from build123d import *

# Parameters (mm, degrees)
SKETCH1_R           = 2.54
BOSS_EXTRUDE1_DEPTH = 3.81
SKETCH2_R           = 4.953
BOSS_EXTRUDE2_DEPTH = 76.2
FILLET1_R           = 2.54


with BuildPart() as part:
    # Sketch1 → Boss-Extrude1 (new body)
    with BuildSketch(Plane(origin=(0, 0, 0), x_dir=(1, 0, 0), z_dir=(0, 1, 0))):
        with BuildLine():
            Line((-13.97, -6.985), (13.97, -6.985))
            ThreePointArc((13.97, -6.985), (15.766051224, -6.241051224), (16.51, -4.445))
            Line((16.51, -4.445), (16.51, 4.445))
            ThreePointArc((16.51, 4.445), (15.766051224, 6.241051224), (13.97, 6.985))
            Line((13.97, 6.985), (-13.97, 6.985))
            ThreePointArc((-13.97, 6.985), (-15.766051224, 6.241051224), (-16.51, 4.445))
            Line((-16.51, 4.445), (-16.51, -4.445))
            ThreePointArc((-16.51, -4.445), (-15.766051224, -6.241051224), (-13.97, -6.985))
        make_face()
        with Locations(Location((-12.7, 0, 0), (0, 0, 90))):
            Circle(SKETCH1_R, mode=Mode.SUBTRACT)
        with Locations(Location((12.7, 0, 0), (0, 0, 90))):
            Circle(SKETCH1_R, mode=Mode.SUBTRACT)
    extrude(amount=BOSS_EXTRUDE1_DEPTH)

    # Sketch2 → Boss-Extrude2 (add)
    with BuildSketch(Plane(origin=(0, 3.81, 0), x_dir=(1, 0, 0), z_dir=(0, 1, 0))):
        with Locations(Location((0, 0, 0), (0, 0, 90))):
            Circle(SKETCH2_R)
    extrude(amount=BOSS_EXTRUDE2_DEPTH)

    # Fillet1
    fillet1_edges = [part.edges().sort_by_distance(p)[0] for p in [
        (0, 3.81, 4.953),
    ]]
    fillet(fillet1_edges, radius=FILLET1_R)


solid = part.part
Verification items for the finished model (mm, model axes). A direction names the side the tool comes from. Coordinates: 2 decimals unless noted, no trailing zeros. Write each loop counter-clockwise with the first axis right and the second up, starting at its lowest first coordinate (ties: lowest second). Pieces come first, ordered by that corner, then holes. Notation, with made-up numbers: M 88.5,7 L 110.5,7 A19 ccw 110.5,35 Z; hole C 77,-9 d5. An arc over 180 degrees is marked long. One line per question, with ' | ' between items.
1) Depth check by flat-ended pin: pin 1 Ø6 at (x, z) = (-12.7, 0) entering from +Y; pin 2 Ø4 at (y, z) = (48.5, 5.5) entering from -X; pin 3 Ø4 at (y, z) = (34, -3.5) entering from -X; pin 4 Ø3 at (x, z) = (12.7, 0) entering from +Y. Enter the tip coordinate at first touch or a pass-through.
Solutions:
pin 1: y = 3.81 | pin 2: x = -3.5 | pin 3: x = -4.72 | pin 4: through
2) Access from +Z, -Z, +X, -X, +Y, -Y to the whole of each face (thin tool, end or side, straight path). Record for faces 4 (the face through (0, 0, 0)), 5 (the face through (-1.488, 42.63, -4.724)).
Solutions:
face 4: +Z, -Z, +X, -X, -Y | face 5: +Y
3) Material ranges on L1, parallel to X at y = 2.6, z = 0; L2, parallel to Z at x = -12.7, y = 1.2 (3 decimals); L3, parallel to Y at x = 7.5, z = -4, recorded low to high.
Solutions:
L1: -16.51 to -15.24, -10.16 to 10.16, 15.24 to 16.51 | L2: -6.985 to -2.54, 2.54 to 6.985 | L3: 0 to 3.81
4) Release check for a two-part mould opening along Z. For faces 1 (the face through (15.18, 1.88, 0.55)), 2 (the face through (0, 2, 6.985)), 3 (the face through (16.51, 2, 0)) record: +Z half, -Z half, draft (parallel to the pull), parting line (faces both ways), or undercut.
Solutions:
face 1: undercut | face 2: +Z half | face 3: draft
5) Sectioned sample at D-D on x = -11.5. Record the cut outline in (y, z) (3 decimals), then the cut area to 3 significant figures.
Solutions:
outline: M 0,-6.985 L 3.81,-6.985 L 3.81,-2.239 L 0,-2.239 Z; M 0,2.239 L 3.81,2.239 L 3.81,6.985 L 0,6.985 Z | area: 36.2 mm^2
6) Sectioned sample at A-A on z = 0. Record the cut outline in (x, y), then the cut area to 3 significant figures.
Solutions:
outline: M -16.51,0 L -15.24,0 L -15.24,3.81 L -16.51,3.81 Z; M -10.16,0 L 10.16,0 L 10.16,3.81 L 7.49,3.81 A2.54 cw 4.95,6.35 L 4.95,80.01 L -4.95,80.01 L -4.95,6.35 A2.54 cw -7.49,3.81 L -10.16,3.81 Z; M 15.24,0 L 16.51,0 L 16.51,3.81 L 15.24,3.81 Z | area: 845 mm^2
7) Sectioned sample at B-B on x = 12.7. Record the cut outline in (y, z) (3 decimals).
Solutions:
outline: M 0,-6.985 L 3.81,-6.985 L 3.81,-2.54 L 0,-2.54 Z; M 0,2.54 L 3.81,2.54 L 3.81,6.985 L 0,6.985 Z
8) Sectioned sample at C-C on y = 67. Record the cut outline in (x, z), then the cut area to 3 significant figures.
Solutions:
outline: C 0,0 d9.91 | area: 77.1 mm^2
